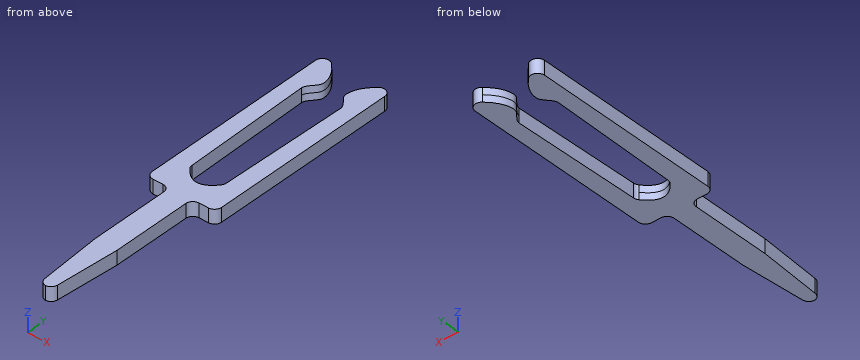
from build123d import *

# Parameters (mm, degrees)
BOSS_EXTRUDE1_DEPTH = 0.2


with BuildPart() as part:
    # Sketch1 → Boss-Extrude1 (new, symmetric)
    with BuildSketch(Plane.XY):
        with BuildLine():
            Line((-0.32, 1.999393664), (-0.32, 4.266775148))
            ThreePointArc((-0.32, 4.266775148), (-0.378578644, 4.408196504), (-0.52, 4.466775148))
            Line((-0.52, 4.466775148), (-0.8, 4.466775148))
            ThreePointArc((-0.8, 4.466775148), (-0.941421356, 4.525353792), (-1, 4.666775148))
            Line((-1, 4.666775148), (-1, 10.057198685))
            ThreePointArc((-1, 10.057198685), (-0.87939743, 10.240763518), (-0.663039519, 10.202944445))
            add(Edge.make_bspline(
                [(-0.663039519, 10.202944445), (-0.487599251, 10.038079386), (-0.326177604, 9.816155039), (-0.310671132, 9.388247389), (-0.548453888, 9.275984696), (-0.567669208, 9.108344969)],
                knots=[0.253308427, 0.253308427, 0.253308427, 0.253308427, 0.663171976, 0.707067436, 1, 1, 1, 1], degree=3))
            Line((-0.567669208, 9.108344969), (-0.495215905, 5.401684718))
            ThreePointArc((-0.495215905, 5.401684718), (-0.483221967, 5.337269967), (-0.451053839, 5.280188217))
            add(Edge.make_bspline(
                [(-0.451053839, 5.280188217), (0, 4.719811783), (0.451053839, 5.280188217)],
                knots=[0.043404734, 0.043404734, 0.043404734, 0.956595266, 0.956595266, 0.956595266], degree=2))
            ThreePointArc((0.451053839, 5.280188217), (0.483221967, 5.337269967), (0.495215905, 5.401684718))
            Line((0.495215905, 5.401684718), (0.567669208, 9.108344969))
            add(Edge.make_bspline(
                [(0.663039519, 10.202944445), (0.487599251, 10.038079386), (0.326177604, 9.816155039), (0.310671132, 9.388247389), (0.548453888, 9.275984696), (0.567669208, 9.108344969)],
                knots=[0.253308427, 0.253308427, 0.253308427, 0.253308427, 0.663171976, 0.707067436, 1, 1, 1, 1], degree=3))
            ThreePointArc((0.663039519, 10.202944445), (0.87939743, 10.240763518), (1, 10.057198685))
            Line((1, 10.057198685), (1, 4.666775148))
            ThreePointArc((1, 4.666775148), (0.941421356, 4.525353792), (0.8, 4.466775148))
            Line((0.8, 4.466775148), (0.52, 4.466775148))
            ThreePointArc((0.52, 4.466775148), (0.378578644, 4.408196504), (0.32, 4.266775148))
            Line((0.32, 4.266775148), (0.32, 1.999393664))
            Line((0.32, 1.999393664), (0.183878151, 0.184435674))
            ThreePointArc((0.183878151, 0.184435674), (0.126073555, 0.058186541), (0, 0))
            ThreePointArc((0, 0), (-0.126073555, 0.058186541), (-0.183878151, 0.184435674))
            Line((-0.183878151, 0.184435674), (-0.32, 1.999393664))
        make_face()
    extrude(amount=BOSS_EXTRUDE1_DEPTH, both=True)


solid = part.part
For this review, take the finished solid that the model builds, in its own axes (mm). Round coordinates to 2 decimals unless told otherwise and drop trailing zeros. Loops run counter-clockwise (first coordinate to the right, second up) from the corner with the lowest first, then second, coordinate; pieces in that order, holes last. Notation, with made-up numbers: (11, -6.5) - (65, -6.5) arc R17 ccw to (65, -1.5) - close; hole circle Ø4 at (-15.5, 37.25). An arc over 180 degrees is marked (long way). One line per item, written item: value. Start each with the question number.
Item 1: Clearance check with a flat-ended pin moving along its axis: pin 1 Ø1 at (x, y) = (-0.5, 3.5) entering from -Z. State where the tip first meets the part, or that it passes through.
Item 2: Take a section at A-A (y = 5.5). Give the boundary of the cut face in (x, z), plus the area to 3 significant figures.
Item 3: Take a section at B-B (y = 2.25). Give the boundary of the cut face in (x, z).
Item 4: For L1, parallel to X at y = 3, z = 0.1; L2, parallel to X at y = 5.75, z = 0; L3, parallel to Y at x = 0.4, z = -0.05, list the stretches that pass through material, from the lowest coordinate up.
Item 5: Take a section at C-C (y = 0.5). Give the boundary of the cut face in (x, z), plus the area to 3 significant figures.
Answer below:
1. pin 1: stops at z = -0.2
2. outline: (-1, -0.2) - (-0.5, -0.2) - (-0.5, 0.2) - (-1, 0.2) - close; (0.5, -0.2) - (1, -0.2) - (1, 0.2) - (0.5, 0.2) - close
2. area: 0.402 mm2
3. outline: (-0.32, -0.2) - (0.32, -0.2) - (0.32, 0.2) - (-0.32, 0.2) - close
4. L1: x = -0.32 to 0.32
4. L2: x = -1 to -0.5, 0.5 to 1
4. L3: y = 4.43 to 5.22, 9.38 to 9.87
5. outline: (-0.21, -0.2) - (0.21, -0.2) - (0.21, 0.2) - (-0.21, 0.2) - close
5. area: 0.166 mm2
